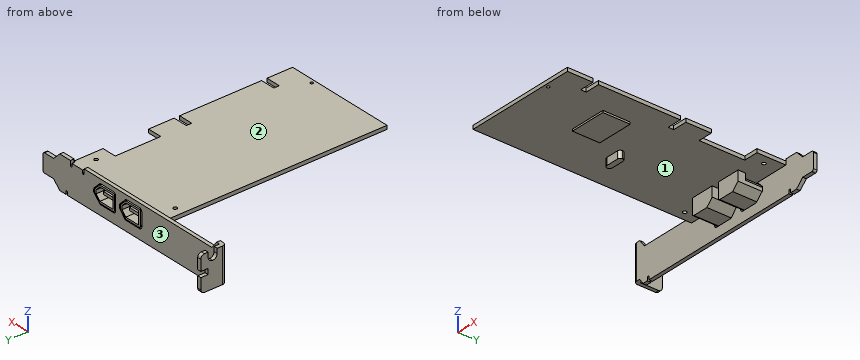
```python
from build123d import *

# Parameters (mm, degrees)
F0_W      = 8
F0_H      = 16
F0_H_2    = 14
F0_H_3    = 45
F1_DEPTH  = 2
F2_W      = 20
F2_H      = 15
F3_DEPTH  = 3
F5_DEPTH  = 4
F6_R      = 0.75
F7_DEPTH  = 25
F8_R      = 1
F9_DEPTH  = 25
F11_DEPTH = 9
F12_SIZE  = 3.5
F13_SIZE  = 3.5
F14_R     = 1
F15_R     = 1
F17_W     = 7
F17_H     = 1.5
F18_DEPTH = 14
F19_DEPTH = 2
F20_W     = 7
F20_H     = 1.5
F21_DEPTH = 14
F22_DEPTH = 2
F24_DEPTH = 9
F26_DEPTH = 9
F29_DEPTH = 2
F31_DEPTH = 12
F32_R     = 2
F33_R     = 2
F34_W     = 4
F34_H     = 3
F35_DEPTH = 25
F37_DEPTH = 25


# Not quite as in the source:
# - two fillets or chamfers of one size are made in one step


with BuildPart() as f1:
    # F0 (on Top) → F1 (new body)
    with BuildSketch(Plane.XY):
        Polygon((22.8202738762, 74.1253000498), (-31.1797261238, 74.1253000498), (-31.1797261238, -45.8746999502), (22.8202738762, -45.8746999502), (22.8202738762, -31.8746999502), (22.8202738762, -28.8746999502), (22.8202738762, 16.1253000498), (22.8202738762, 19.1253000498), (22.8202738762, 33.1253000498), (22.8202738762, 58.1253000498), align=None)
        with Locations((26.8202738762, 66.1253000498)):
            Rectangle(F0_W, F0_H)
        with Locations((26.8202738762, -38.8746999502)):
            Rectangle(F0_W, F0_H_2)
        with Locations((26.8202738762, 26.1253000498)):
            Rectangle(F0_W, F0_H_2)
        with Locations((26.8202738762, -6.3746999502)):
            Rectangle(F0_W, F0_H_3)
    extrude(amount=F1_DEPTH)

    # F2 (on face) → F3 (join)
    with BuildSketch(Plane.XY.offset(2)):
        with Locations((5.8202738762, -6.3746999502)):
            Rectangle(F2_W, F2_H)
    extrude(amount=-F3_DEPTH)

    # F4 (on face) → F5 (join)
    with BuildSketch(Plane(origin=(0, 0, 0), x_dir=(1, 0, 0), z_dir=(0, 0, -1))):
        with BuildLine():
            ThreePointArc((-4.1797261238, -13.6253000498), (-4.619065952, -12.564639878), (-5.6797261238, -12.1253000498))
            Line((-5.6797261238, -12.1253000498), (-12.6797261238, -12.1253000498))
            ThreePointArc((-12.6797261238, -12.1253000498), (-13.7403862956, -12.564639878), (-14.1797261238, -13.6253000498))
            ThreePointArc((-14.1797261238, -13.6253000498), (-13.7403862956, -14.6859602216), (-12.6797261238, -15.1253000498))
            Line((-12.6797261238, -15.1253000498), (-5.6797261238, -15.1253000498))
            ThreePointArc((-5.6797261238, -15.1253000498), (-4.619065952, -14.6859602216), (-4.1797261238, -13.6253000498))
        make_face()
    extrude(amount=F5_DEPTH)

    # F6 (on face) → F7 (cut)
    with BuildSketch(Plane(origin=(0, 0, 0), x_dir=(1, 0, 0), z_dir=(0, 0, -1))):
        with Locations((15.8202738762, 43.8746999502)):
            Circle(F6_R)
    extrude(amount=-F7_DEPTH, mode=Mode.SUBTRACT)

    # F8 (on face) → F9 (cut)
    with BuildSketch(Plane(origin=(0, 0, 0), x_dir=(1, 0, 0), z_dir=(0, 0, -1))):
        with Locations((25.8202738762, -66.1253000498)):
            Circle(F8_R)
        with Locations((-26.1797261238, -66.1253000498)):
            Circle(F8_R)
    extrude(amount=-F9_DEPTH, mode=Mode.SUBTRACT)

    # F10 (on face) → F11 (join)
    with BuildSketch(Plane(origin=(0, 0, 0), x_dir=(1, 0, 0), z_dir=(0, 0, -1))):
        Polygon((14.8202738762, -76.1253000498), (14.8202738762, -74.1253000498), (14.8202738762, -61.1253000498), (1.8202738762, -61.1253000498), (1.8202738762, -74.1253000498), (1.8202738762, -76.1253000498), align=None)
        Polygon((-15.1797261238, -61.1253000498), (-15.1797261238, -74.1253000498), (-15.1797261238, -76.1253000498), (-2.1797261238, -76.1253000498), (-2.1797261238, -74.1253000498), (-2.1797261238, -61.1253000498), align=None)
    extrude(amount=F11_DEPTH)

    # F12
    f12_edges = [f1.edges().sort_by_distance(p)[0] for p in [
        (14.820274, 68.6253, -9),
    ]]
    chamfer(f12_edges, length=F12_SIZE)

    # F13
    f13_edges = [f1.edges().sort_by_distance(p)[0] for p in [
        (14.820274, 75.1253, 0),
        (-2.179726, 75.1253, 0),
        (-2.179726, 68.6253, -9),
    ]]
    chamfer(f13_edges, length=F13_SIZE)

    # F14
    f14_edges = [f1.edges().sort_by_distance(p)[0] for p in [
        (1.820274, 68.6253, -9),
    ]]
    fillet(f14_edges, radius=F14_R)

    # F15
    f15_edges = [f1.edges().sort_by_distance(p)[0] for p in [
        (-15.179726, 68.6253, -9),
    ]]
    fillet(f15_edges, radius=F15_R)

    # F17 (on face) → F18 (cut)
    with BuildSketch(Plane(origin=(0, 76.1253000498, 0), x_dir=(-1, 0, 0), z_dir=(0, 1, 0))):
        Polygon((14.1797261238, -8), (14.1797261238, -1), (5.6797261238, -1), (3.1797261238, -3.5), (3.1797261238, -5.5), (5.6797261238, -8), align=None)
        with Locations((9.1797261238, -4.75)):
            Rectangle(F17_W, F17_H, mode=Mode.SUBTRACT)
    extrude(amount=-F18_DEPTH, mode=Mode.SUBTRACT)

    # F19 (cut): a face of the model
    f19_faces = [f1.faces().sort_by_distance(p)[0] for p in [
        (-9.1797261238, 76.1253000498, -4.75),
    ]]
    extrude(f19_faces, amount=-F19_DEPTH, mode=Mode.SUBTRACT)

    # F20 (on face) → F21 (cut)
    with BuildSketch(Plane(origin=(0, 76.1253000498, 0), x_dir=(-1, 0, 0), z_dir=(0, 1, 0))):
        Polygon((-2.8202738762, -8), (-2.8202738762, -4), (-2.8202738762, -1), (-11.3202738762, -1), (-13.8202738762, -3.5), (-13.8202738762, -5.5), (-11.3202738762, -8), align=None)
        with Locations((-7.8202738762, -4.75)):
            Rectangle(F20_W, F20_H, mode=Mode.SUBTRACT)
    extrude(amount=-F21_DEPTH, mode=Mode.SUBTRACT)

    # F22 (cut): a face of the model
    f22_faces = [f1.faces().sort_by_distance(p)[0] for p in [
        (7.8202738762, 76.1253000498, -4.75),
    ]]
    extrude(f22_faces, amount=-F22_DEPTH, mode=Mode.SUBTRACT)

    # F23 (on face) → F24 (cut)
    with BuildSketch(Plane(origin=(0, 74.1253000498, 0), x_dir=(-1, 0, 0), z_dir=(0, 1, 0))):
        Polygon((-11.3202738762, 0), (-14.8202738762, 0), (-14.8202738762, -3.5), align=None)
    extrude(amount=-F24_DEPTH, mode=Mode.SUBTRACT)

    # F25 (on face) → F26 (cut)
    with BuildSketch(Plane(origin=(0, 74.1253000498, 0), x_dir=(-1, 0, 0), z_dir=(0, 1, 0))):
        Polygon((2.1797261238, -3.5), (5.6797261238, 0), (2.1797261238, 0), align=None)
    extrude(amount=-F26_DEPTH, mode=Mode.SUBTRACT)

    # F28 (on offset) → F29 (join)
    with BuildSketch(Plane.XZ.offset(-76)):
        with BuildLine():
            Line((21.8447855255, 3), (1.8447855255, 3))
            Line((1.8447855255, 3), (0, 3))
            Line((0, 3), (-62.1552144745, 3))
            Line((-62.1552144745, 3), (-65.1552144745, 7))
            Line((-65.1552144745, 7), (-69.1552144745, 7))
            Line((-69.1552144745, 7), (-69.1552144745, -4.8977956176))
            Line((-69.1552144745, -4.8977956176), (-69.1552144745, -12))
            Line((-69.1552144745, -12), (-65.1552144745, -12))
            Line((-65.1552144745, -12), (-63.1552144745, -15))
            Line((-63.1552144745, -15), (-60.1552144745, -15))
            Line((-60.1552144745, -15), (-60.1552144745, -13.5))
            ThreePointArc((-60.1552144745, -13.5), (-60.0087678651, -13.1464466094), (-59.6552144745, -13))
            ThreePointArc((-59.6552144745, -13), (-59.3016610839, -13.1464466094), (-59.1552144745, -13.5))
            Line((-59.1552144745, -13.5), (-59.1552144745, -15))
            Line((-59.1552144745, -15), (32.8447855255, -15))
            Line((32.8447855255, -15), (32.8447855255, -13.5))
            ThreePointArc((32.8447855255, -13.5), (32.9912321349, -13.1464466094), (33.3447855255, -13))
            ThreePointArc((33.3447855255, -13), (33.6983389161, -13.1464466094), (33.8447855255, -13.5))
            Line((33.8447855255, -13.5), (33.8447855255, -15))
            Line((33.8447855255, -15), (37.8447855255, -15))
            Line((37.8447855255, -15), (41.8670170307, -11.0439766385))
            Line((41.8670170307, -11.0439766385), (47.8670170307, -11.0439766385))
            ThreePointArc((47.8670170307, -11.0439766385), (48.5741238119, -10.7510834197), (48.8670170307, -10.0439766385))
            Line((48.8670170307, -10.0439766385), (48.8670170307, -6.0439766385))
            Line((48.8670170307, -6.0439766385), (48.8670170307, -2.0439766385))
            ThreePointArc((48.8670170307, -2.0439766385), (48.5741238119, -1.3368698573), (47.8670170307, -1.0439766385))
            Line((47.8670170307, -1.0439766385), (41.8670170307, -1.0439766385))
            Line((41.8670170307, -1.0439766385), (37.8447855255, 3))
            Line((37.8447855255, 3), (30.8447855255, 3))
            Line((30.8447855255, 3), (30.8447855255, 0.5))
            ThreePointArc((30.8447855255, 0.5), (30.6983389161, 0.1464466094), (30.3447855255, 0))
            ThreePointArc((30.3447855255, 0), (29.9912321349, 0.1464466094), (29.8447855255, 0.5))
            Line((29.8447855255, 0.5), (29.8447855255, 2))
            Line((29.8447855255, 2), (22.8447855255, 2))
            Line((22.8447855255, 2), (22.8447855255, 0.5))
            ThreePointArc((22.8447855255, 0.5), (22.6983389161, 0.1464466094), (22.3447855255, 0))
            ThreePointArc((22.3447855255, 0), (21.9912321349, 0.1464466094), (21.8447855255, 0.5))
            Line((21.8447855255, 0.5), (21.8447855255, 3))
        make_face()
        with BuildLine():
            Line((-5.1067974085, -9.6197371359), (-9.916828014, -9.6487514675))
            Line((-9.916828014, -9.6487514675), (-14.5359628499, -9.6487514675))
            ThreePointArc((-14.5359628499, -9.6487514675), (-15.5966230216, -9.2094116392), (-16.0359628499, -8.1487514675))
            Line((-16.0359628499, -8.1487514675), (-16.0359628499, -4.194740206))
            Line((-16.0359628499, -4.194740206), (-16.0359628499, -0.8))
            ThreePointArc((-16.0359628499, -0.8), (-15.5966230216, 0.2606601718), (-14.5359628499, 0.7))
            Line((-14.5359628499, 0.7), (-9.4512412325, 0.7))
            Line((-9.4512412325, 0.7), (-5.5935280398, 0.7))
            Line((-5.5935280398, 0.7), (-1.5013976704, -3.5296175629))
            Line((-1.5013976704, -3.5296175629), (-1.5013976704, -5.5249878205))
            Line((-1.5013976704, -5.5249878205), (-5.1067974085, -9.6197371359))
        make_face(mode=Mode.SUBTRACT)
        with BuildLine():
            Line((15.5488683626, -5.5253235623), (11.2658282742, -9.6197371359))
            Line((11.2658282742, -9.6197371359), (2.5931737488, -9.6197371359))
            ThreePointArc((2.5931737488, -9.6197371359), (1.532513577, -9.1803973077), (1.0931737488, -8.1197371359))
            Line((1.0931737488, -8.1197371359), (1.0931737488, -4.0044868365))
            Line((1.0931737488, -4.0044868365), (1.0931737488, -0.8))
            ThreePointArc((1.0931737488, -0.8), (1.532513577, 0.2606601718), (2.5931737488, 0.7))
            Line((2.5931737488, 0.7), (7.3360428214, 0.7))
            Line((7.3360428214, 0.7), (11.4213749766, 0.7))
            Line((11.4213749766, 0.7), (15.5199731484, -3.473744262))
            Line((15.5199731484, -3.473744262), (15.5488683626, -5.5253235623))
        make_face(mode=Mode.SUBTRACT)
    extrude(amount=F29_DEPTH)

    # F30 (on face) → F31 (join)
    with BuildSketch(Plane(origin=(0, 76, 0), x_dir=(-1, 0, 0), z_dir=(0, 1, 0))):
        Polygon((67.1552144745, 7), (67.1552144745, -5.6737242267), (67.1552144745, -12), (69.1552144745, -12), (69.1552144745, 7), align=None)
    extrude(amount=F31_DEPTH)

    # F32
    f32_edges = [f1.edges().sort_by_distance(p)[0] for p in [
        (-68.155214, 88, -12),
        (-68.155214, 88, 7),
    ]]
    fillet(f32_edges, radius=F32_R)

    # F33
    f33_edges = [f1.edges().sort_by_distance(p)[0] for p in [
        (-69.155214, 74, -2.5),
    ]]
    fillet(f33_edges, radius=F33_R)

    # F34 (on face) → F35 (cut)
    with BuildSketch(Plane(origin=(-69.1552144745, 0, 0), x_dir=(0, -1, 0), z_dir=(-1, 0, 0))):
        with Locations((-86, -2.5)):
            Rectangle(F34_W, F34_H)
    extrude(amount=-F35_DEPTH, mode=Mode.SUBTRACT)

    # F36 (on face) → F37 (cut)
    with BuildSketch(Plane(origin=(-69.1552144745, 0, 0), x_dir=(0, -1, 0), z_dir=(-1, 0, 0))):
        with BuildLine():
            Line((-79, 7), (-84, 7))
            Line((-84, 7), (-84, 4.5))
            ThreePointArc((-84, 4.5), (-83.267766953, 2.732233047), (-81.5, 2))
            ThreePointArc((-81.5, 2), (-79.732233047, 2.732233047), (-79, 4.5))
            Line((-79, 4.5), (-79, 7))
        make_face()
    extrude(amount=-F37_DEPTH, mode=Mode.SUBTRACT)


solid = f1.part
```
CAD build for the part. Positions are in the model's coordinates, mm. Face numbers are marked on the shaded views. Coordinates: 2 decimals unless noted, no trailing zeros. Order: outer loops, then holes, each group sorted by start corner. A loop starts at its lowest first (then second) coordinate and runs counter-clockwise, first axis right, second up. Notation, with made-up numbers: M 14.25,5.25 L 25.25,5.25 A24 ccw 25.25,40.25 Z; hole C 20.5,-31 d3. An arc over 180 degrees is marked long. Write each question's results on one line, items separated by ' | '. Start each with the question number.
Q1. Drill centre lines: probe 1 along Y at (x, z) = (-6.5, -3.5); probe 2 along Y at (x, z) = (27.5, 0.5); probe 3 along Z at (x, y) = (-7.5, -18.5). Where is each one in solid material? Low to high. Write a range as from..to.
Q2. Flat gauge pins, fed straight in: P1, Ø5, axis at y = 25, z = 0, coming from the -X side; P2, Ø0.9, axis at x = -9.5, y = 13.5, coming from the -Z side; P3, Ø0.8, axis at x = 30, z = 1, coming from the +Y side. Where does each tip first touch, or does it go through?
Q3. Cut at B-B (x = -29.5). List the corners of the cut face in (y, z).
Q4. Cut at A-A (y = -7.5). List the corners of the cut face in (x, z).
Q5. Cut at C-C (y = 47.5). List the corners of the cut face in (x, z).
Q6. Cut at D-D (y = 26.5). List the corners of the cut face in (x, z), then the cut area to 3 significant figures.
Q7. Pull direction Y, two halves, no side cores. Call the marked faces 1, 2 and 3: +Y half, -Y half, draft (parallel to the pull), parting line (faces both ways), or undercut.
Found:
1) probe 1: 12.13..15.13, 61.13..62.13 | probe 2: -45.87..-31.87, -28.87..16.13, 19.13..33.13, 58.13..76 | probe 3: 0..2
2) P1: x = -31.18 | P2: z = -4 | P3: y = 76
3) outline: M -45.87,0 L 74,0 L 74,-15 L 76,-15 L 76,3 L 74,3 L 74,2 L -45.87,2 Z
4) outline: M -31.18,0 L -4.18,0 L -4.18,-1 L 15.82,-1 L 15.82,0 L 30.82,0 L 30.82,2 L -31.18,2 Z
5) outline: M -31.18,0 L 22.82,0 L 22.82,2 L -31.18,2 Z
6) outline: M -31.18,0 L 30.82,0 L 30.82,2 L -31.18,2 Z | area: 124 mm²
7) face 1: undercut | face 2: draft | face 3: +Y half
